Part model, mm, in its own coordinate system. A direction names the side the tool comes from. Give positions to 0.01 mm unless a question says otherwise; leave off trailing zeros. Loops run counter-clockwise (first coordinate to the right, second up) from the corner with the lowest first, then second, coordinate; pieces in that order, holes last. Notation, with made-up numbers: M -21.75,75.25 L 17.25,75.25 A22 cw 17.25,107.25 Z; hole C 84.5,13.25 d7. An arc over 180 degrees is marked long. Answer in a Markdown table with one row per item.
from build123d import *

# Parameters (mm, degrees)
SKETCH1_W           = 152.4
SKETCH1_H           = 76.2
BOSS_EXTRUDE1_DEPTH = 31.75
SKETCH2_R           = 17.145
CUT_EXTRUDE1_DEPTH  = 174.321269612
SKETCH2_2_R         = 25.4
SKETCH2_2_R_2       = 17.145
CUT_EXTRUDE3_DEPTH  = 12.446
SKETCH3_R           = 3.175
CUT_EXTRUDE4_DEPTH  = 31.75


with BuildPart() as part:
    # Sketch1 → Boss-Extrude1 (new body)
    with BuildSketch(Plane.XY):
        with Locations((76.2, 38.1)):
            Rectangle(SKETCH1_W, SKETCH1_H)
    extrude(amount=BOSS_EXTRUDE1_DEPTH)

    # Sketch2 → Cut-Extrude1 (cut, through all)
    with BuildSketch(Plane(origin=(0, 0, 0), x_dir=(-1, 0, 0), z_dir=(0, 0, -1))):
        with Locations((-76.2, 38.1)):
            Circle(SKETCH2_R)
    extrude(amount=-CUT_EXTRUDE1_DEPTH, mode=Mode.SUBTRACT)

    # Sketch2_2 → Cut-Extrude3 (cut)
    with BuildSketch(Plane(origin=(0, 0, 0), x_dir=(-1, 0, 0), z_dir=(0, 0, -1))):
        with Locations((-76.2, 38.1)):
            Circle(SKETCH2_2_R)
        with Locations((-76.2, 38.1)):
            Circle(SKETCH2_2_R_2, mode=Mode.SUBTRACT)
    cut_extrude3 = extrude(amount=-CUT_EXTRUDE3_DEPTH, mode=Mode.SUBTRACT)

    # Mirror2: Cut-Extrude3 across plane
    add(cut_extrude3.mirror(Plane(origin=(0, 0, 15.875), x_dir=(1, 0, 0), z_dir=(0, 0, -1))), mode=Mode.SUBTRACT)

    # Sketch3 → Cut-Extrude4 (cut)
    with BuildSketch(Plane(origin=(152.4, 0, 0), x_dir=(0, 0, -1), z_dir=(1, 0, 0))):
        with Locations(Location((-15.875, 57.15, 0), (0, 0, 90))):
            Circle(SKETCH3_R)
        with Locations(Location((-15.875, 19.05, 0), (0, 0, 90))):
            Circle(SKETCH3_R)
        with Locations(Location((-15.875, 38.1, 0), (0, 0, 90))):
            Circle(SKETCH3_R)
    extrude(amount=-CUT_EXTRUDE4_DEPTH, mode=Mode.SUBTRACT)


solid = part.part
(1) Drill centre lines: line 1 along Y through (x, z) = (76, 8); line 2 along X through (y, z) = (38.5, 21.5); line 3 along X through (y, z) = (38, 14). Where is each one in solid material? Low to high.
Recorded:
| item | result |
|---|---|
| line 1 | y = 0 to 12.7, 63.5 to 76.2 |
| line 2 | x = 0 to 50.8, 101.6 to 152.4 |
| line 3 | x = 0 to 59.06, 93.34 to 120.65 |
(2) Saw through at B-B (x = 76.2). Write the cut outline in (y, z) (3 decimals).
Recorded:
| item | result |
|---|---|
| outline | M 0,0 L 12.7,0 L 12.7,12.446 L 20.955,12.446 L 20.955,19.304 L 12.7,19.304 L 12.7,31.75 L 0,31.75 Z; M 55.245,12.446 L 63.5,12.446 L 63.5,0 L 76.2,0 L 76.2,31.75 L 63.5,31.75 L 63.5,19.304 L 55.245,19.304 Z |
(3) Pull direction Z, two halves, no side cores. Call faces 1 (the face through (75, 0, 16)), 2 (the face through (70.9, 21.5, 19.304)), 3 (the face through (136.747, 34.928, 16.015)): +Z half, -Z half, draft (parallel to the pull), parting line (faces both ways), or undercut.
Recorded:
| item | result |
|---|---|
| face 1 | draft |
| face 2 | +Z half |
| face 3 | undercut |
(4) Pin check, flat tips, straight feed: pin 1 Ø4 at (y, z) = (38.1, 15.875) entering from +X; pin 2 Ø3 at (x, y) = (60, 30) entering from -Z. Stop position of each tip, or through.
Recorded:
| item | result |
|---|---|
| pin 1 | stops at x = 120.65 |
| pin 2 | stops at z = 12.45 |
(5) Saw through at A-A (y = 38.1). Write the cut outline in (x, z) (3 decimals), plus the area to 3 significant figures.
Recorded:
| item | result |
|---|---|
| outline | M 0,0 L 50.8,0 L 50.8,12.446 L 59.055,12.446 L 59.055,19.304 L 50.8,19.304 L 50.8,31.75 L 0,31.75 Z; M 93.345,12.446 L 101.6,12.446 L 101.6,0 L 152.4,0 L 152.4,12.7 L 120.65,12.7 L 120.65,19.05 L 152.4,19.05 L 152.4,31.75 L 101.6,31.75 L 101.6,19.304 L 93.345,19.304 Z |
| area | 3,140 mm^2 |
(6) Saw through at C-C (z = 25). Write the cut outline in (x, y).
Recorded:
| item | result |
|---|---|
| outline | M 0,0 L 152.4,0 L 152.4,76.2 L 0,76.2 Z; hole C 76.2,38.1 d50.8 |
(7) Saw through at D-D (x = 137.5). Write the cut outline in (y, z) (3 decimals).
Recorded:
| item | result |
|---|---|
| outline | M 0,0 L 76.2,0 L 76.2,31.75 L 0,31.75 Z; hole C 19.05,15.875 d6.35; hole C 38.1,15.875 d6.35; hole C 57.15,15.875 d6.35 |
(8) Which spindle directions (+Z, -Z, +X, -X, +Y, -Y) get a long thin tool onto all of the face, cutting with end or side? Do faces 4 (the face through (120.65, 38, 16)), 5 (the face through (96.357, 22.644, 6.136)), 6 (the face through (96.357, 22.644, 25.614)), 7 (the face through (75, 64, 0)). Say none if no direction does.
Recorded:
| item | result |
|---|---|
| face 4 | +X |
| face 5 | -Z |
| face 6 | +Z |
| face 7 | -Z, +X, -X, +Y, -Y |
